Job drawing, mm, ordinate dimensions from the low corner. One solid piece. Give positions to 0.01 mm unless a question says otherwise; leave off trailing zeros. Write each loop counter-clockwise with the first axis right and the second up, starting at its lowest first coordinate (ties: lowest second). Pieces come first, ordered by that corner, then holes. Notation, with made-up numbers: M 21.25,59 L 40.25,59 A24 cw 40.25,80 Z; hole C 19,35.5 d2. An arc over 180 degrees is marked long. Use CSV: the item, a comma, the result in double quotes. Start each with the question number.
Item 1: Cut at A-A (y = 3.05). List the corners of the cut face in (x, z), then the cut area to 3 significant figures.
Item 2: Pin check, flat tips, straight feed: pin 1 (2 mm diameter, centred on x = 55, z = 120, fed in from -Y); pin 2 (3 mm diameter, centred on x = 125, z = 128, fed in from +Y). Stop position of each tip, or through.
Item 3: Cut at B-B (x = 36). List the corners of the cut face in (y, z).
Item 4: Drill centre lines: line 1 (Z direction, x = 125, y = 3.1); line 2 (Z direction, x = 44.5, y = 4.1); line 3 (Z direction, x = 55, y = 1.5). Where is each one in solid material? Low to high. Write a range as [from, to].
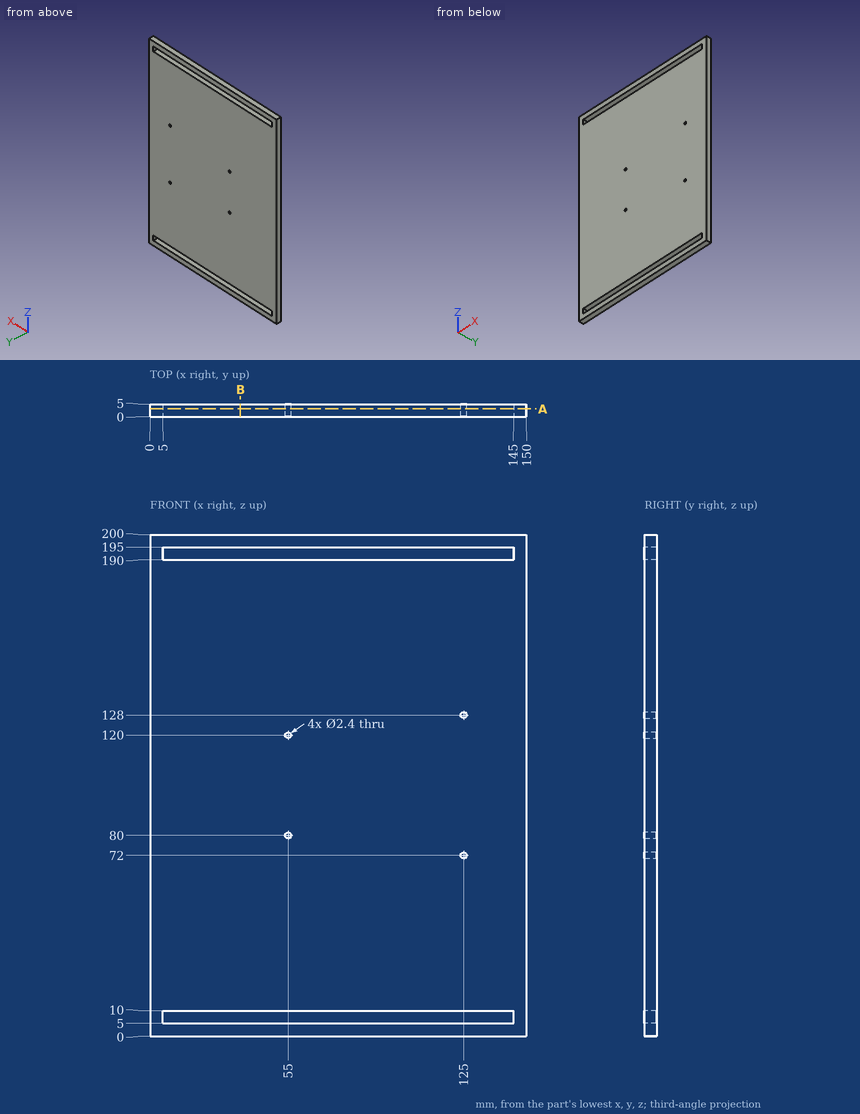
Worked answers:
1,outline,"M 0,0 L 150,0 L 150,200 L 0,200 Z; hole M 5,5 L 145,5 L 145,10 L 5,10 Z; hole M 5,190 L 145,190 L 145,195 L 5,195 Z; hole C 55,80 d2.4; hole C 55,120 d2.4; hole C 125,72 d2.4; hole C 125,128 d2.4"
1,area,"28,600 mm^2"
2,pin 1,"passes through"
2,pin 2,"stops at y = 5"
3,outline,"M 0,0 L 5,0 L 5,5 L 0,5 Z; M 0,10 L 5,10 L 5,190 L 0,190 Z; M 0,195 L 5,195 L 5,200 L 0,200 Z"
4,line 1,"z = [0, 5], [10, 70.8], [73.2, 126.8], [129.2, 190], [195, 200]"
4,line 2,"z = [0, 5], [10, 190], [195, 200]"
4,line 3,"z = [0, 5], [10, 78.8], [81.2, 118.8], [121.2, 190], [195, 200]"
